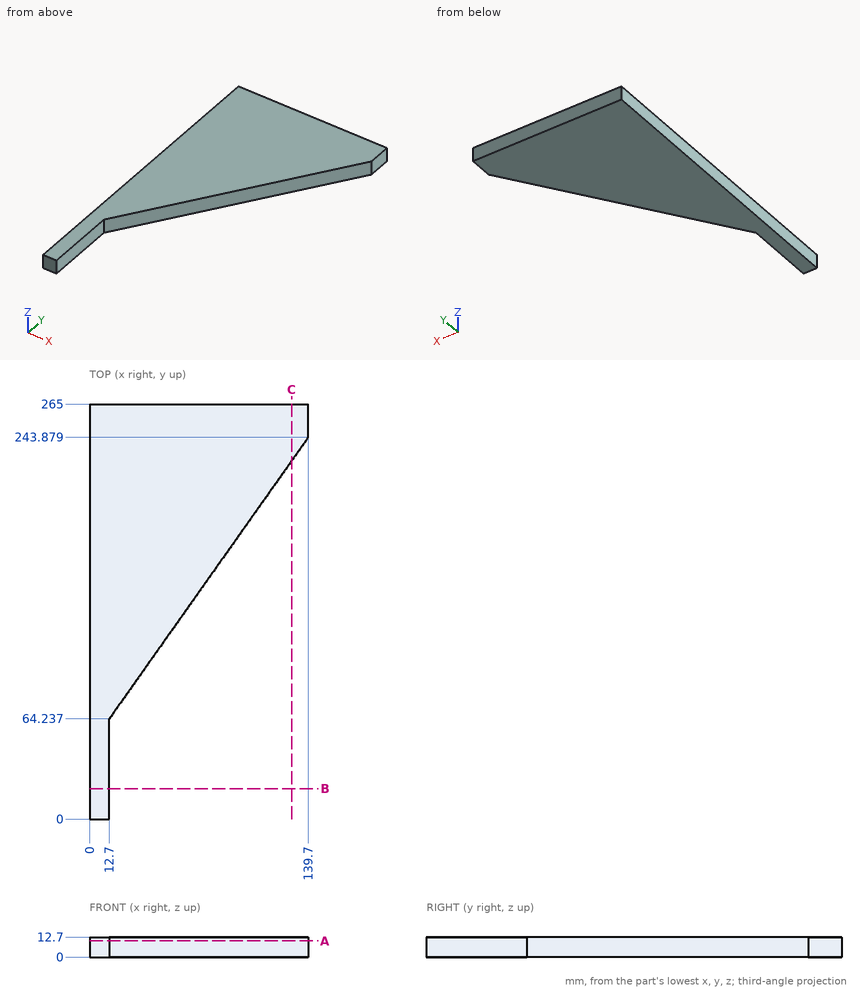
Drawing for the job (mm, zero at the part's lowest x, y, z). Round coordinates to 2 decimals unless told otherwise and drop trailing zeros. Loops run counter-clockwise (first coordinate to the right, second up) from the corner with the lowest first, then second, coordinate; pieces in that order, holes last. Notation, with made-up numbers: M -7.75,-4.75 L 49.25,-4.75 A29 cw 49.25,20.25 Z; hole C -10.5,52.5 d10. An arc over 180 degrees is marked long. Use a Markdown table: item, result. Add a question column.
(1) Cut at B-B (y = 19.5). Give the cut face in (x, z), and give its area (3 significant figures).
(2) Cut at C-C (x = 129). Give the cut face in (y, z).
(3) Cut at A-A (z = 10.25). Give the cut face in (x, y), and give its area (3 significant figures).
(4) Flat gauge pins, fed straight in: pin 1 (1.5 mm diameter, centred on x = 45.5, z = 11, fed in from -Y); pin 2 (3 mm diameter, centred on x = 122.5, z = 9.5, fed in from -Y); pin 3 (5 mm diameter, centred on y = 96, z = 5, fed in from +X). Where does each tip first touch, or does it go through?
(5) Drill centre lines: line 1 (X direction, y = 42.5, z = 2.5); line 2 (X direction, y = 86, z = 5.5) (1 decimal); line 3 (Y direction, x = 72.5, z = 3.5) (1 decimal). Where is each one in solid material? Low to high.
Geometry says:
| question | item | result |
|---|---|---|
| 1 | outline | M 0,0 L 12.7,0 L 12.7,12.7 L 0,12.7 Z |
| 1 | area | 161 mm² |
| 2 | outline | M 228.74,0 L 265,0 L 265,12.7 L 228.74,12.7 Z |
| 3 | outline | M 0,0 L 12.7,0 L 12.7,64.24 L 139.7,243.88 L 139.7,265 L 0,265 Z |
| 3 | area | 17,500 mm² |
| 4 | pin 1 | stops at y = 109.57 |
| 4 | pin 2 | stops at y = 217.43 |
| 4 | pin 3 | stops at x = 36.92 |
| 5 | line 1 | x = 0 to 12.7 |
| 5 | line 2 | x = 0 to 28.1 |
| 5 | line 3 | y = 148.8 to 265 |
